```python
from build123d import *

# Parameters (mm, degrees)
BOSS_EXTRU_1_DEPTH = 3


with BuildPart() as part:
    # Esquisse1 → Boss.-Extru.1 (new body)
    with BuildSketch(Plane(origin=(0, 0, 0), x_dir=(1, 0, 0), z_dir=(0, 1, 0))):
        Polygon((0, 0), (0, 86.036465453), (9.829824531, 79.153548216), (8.109095222, 76.696092084), (16.300615665, 70.96032772), (18.021344974, 73.417783853), (26.212865417, 67.682019489), (24.492136108, 65.224563357), (32.683656551, 59.488798993), (34.40438586, 61.946255126), (42.595906303, 56.210490762), (40.875176994, 53.75303463), (49.066697437, 48.017270266), (50.787426746, 50.474726399), (58.978947189, 44.738962035), (57.25821788, 42.281505903), (65.449738323, 36.545741539), (67.170467632, 39.003197672), (75.361988075, 33.267433308), (73.641258766, 30.809977175), (81.832779208, 25.074212812), (83.553508517, 27.531668945), (91.74502896, 21.795904581), (90.024299651, 19.338448448), (98.215820094, 13.602684085), (99.936549403, 16.060140218), (108.128069846, 10.324375854), (106.407340537, 7.866919721), (114.59886098, 2.131155358), (116.319590289, 4.588611491), (122.872806643, 0), (122.872806643, -25), (110, -25), (110, -22), (100, -22), (100, -25), (90, -25), (90, -22), (80, -22), (80, -25), (70, -25), (70, -22), (60, -22), (60, -25), (50, -25), (50, -22), (40, -22), (40, -25), (30, -25), (30, -22), (20, -22), (20, -25), (10, -25), (10, -22), (0, -22), align=None)
    extrude(amount=BOSS_EXTRU_1_DEPTH)


solid = part.part
```
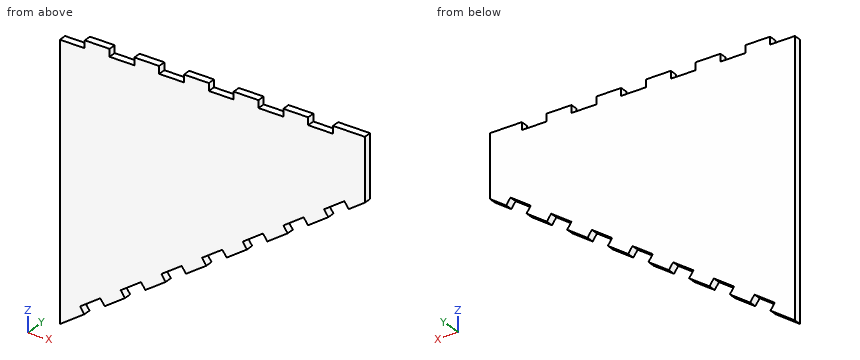
CAD build for the part. Positions are in the model's coordinates, mm. Give positions to 0.01 mm unless a question says otherwise; leave off trailing zeros. Order: outer loops, then holes, each group sorted by start corner. A loop starts at its lowest first (then second) coordinate and runs counter-clockwise, first axis right, second up.
(1) Saw through at B-B, the plane x = 44.5. Give the cut face in (y, z).
(2) Flat gauge pins, fed straight in: pin 1 (1.5 mm diameter, centred on x = 106, y = 1.5, fed in from +Z); pin 2 (0.9 mm diameter, centred on y = 1, z = 24, fed in from -X). Where does each tip first touch, or does it go through?
(3) Saw through at A-A, the plane x = 85. Give the cut face in (y, z).
(4) Drill centre lines: L1, parallel to X at y = 0.9, z = -15.5; L2, parallel to Z at x = 74.5, y = 1.75; L3, parallel to X at y = 2.6, z = -14. Where is each one in solid material? Low to high.
Results found:
1. outline: (0, -51.21) - (3, -51.21) - (3, 22) - (0, 22) - close
2. pin 1: stops at z = 22
2. pin 2: stops at x = 10
3. outline: (0, -26.52) - (3, -26.52) - (3, 22) - (0, 22) - close
4. L1: x = 0 to 95.51, 99.54 to 100.74
4. L2: z = -33.87 to -32.04, -30.21 to 25
4. L3: x = 0 to 97.65, 98.49 to 102.88
